The model under review builds one solid part; all positions refer to its coordinate system, in mm. A direction names the side the tool comes from. Round coordinates to 2 decimals unless told otherwise and drop trailing zeros. Write each loop counter-clockwise with the first axis right and the second up, starting at its lowest first coordinate (ties: lowest second). Pieces come first, ordered by that corner, then holes. Notation, with made-up numbers: (43.25, 26) -> (80.25, 26) arc R17 ccw to (80.25, 41) -> close; hole circle Ø3 at (21.25, -29.75). An arc over 180 degrees is marked (long way). Return JSON: item names as keys, results as strings. Group by question number.
1. Mouldability with a two-part tool opening along X and no side actions: class faces 1 (the flat face through (-3, -52, 0)), 2 (the cylindrical face through (47.69, -15.02, 24.65)), 3 (the cylindrical face through (619.984, 195.242, 747.325)) as pulls with the +X half, pulls with the -X half, needs draft (parallel to the pull), parting line crosses it, or undercut.
2. Take a section at C-C, the plane y = 0. Write out the cut boundary in (x, z), then the cut area to 3 significant figures.
3. Take a section at D-D, the plane x = -296. Write out the cut boundary in (y, z).
4. Tool access review of faces 4 (the cylindrical face through (49.205, 49.788, 747.675)), 5 (the flat face through (-88, 130, 388)), 6 (the flat face through (110, -2, 388)), 7 (the flat face through (-130, -2, 388)), 8 (the flat face through (130, -2, 388)): name each direction out of +Z, -Z, +X, -X, +Y, -Y from which nothing blocks a thin tool from reaching the whole face with its end or side.
5. Clearance check with flat-ended pins moving along their axes: P1, Ø1, axis at x = -305, y = 193.5, coming from the -Z side; P2, Ø7.5, axis at x = 88.5, z = 749, coming from the +Y side; P3, Ø7.5, axis at y = 77.5, z = 750.5, coming from the -X side. State where each tip first meets the part, or that it passes through.
6. For line 1 along Y through (x, z) = (0, 10); line 2 along X through (y, z) = (-61, 473.5), list the stretches that pass through material, from the lowest coordinate up. Write a range as from..to.
7. Take a section at A-A, the plane z = 598. Write out the cut boundary in (x, y), then the cut area to 3 significant figures.
8. Take a section at B-B, the plane x = 0. Write out the cut boundary in (y, z).
from build123d import *

# Parameters (mm, degrees)
F0_R      = 250
F1_DEPTH  = 50
F2_R      = 30
F3_W      = 260
F3_H      = 260
F3_W_2    = 220
F3_H_2    = 220
F4_DEPTH  = 685
F5_R      = 650
F5_W      = 260
F5_H      = 260
F5_W_2    = 220
F5_H_2    = 220
F6_DEPTH  = 25
F8_DEPTH  = 100
F9_W      = 160
F9_H      = 585
F10_DEPTH = 40
F11_R     = 50
F12_DEPTH = 50


with BuildPart() as f1:
    # F0 (on Top) → F1 (new body)
    with BuildSketch(Plane.XY):
        Circle(F0_R)
    extrude(amount=F1_DEPTH)

    # F2
    f2_edges = [f1.edges().sort_by_distance(p)[0] for p in [
        (-250, 0, 50),
    ]]
    fillet(f2_edges, radius=F2_R)

    # F3 (on face) → F4 (join)
    with BuildSketch(Plane.XY.offset(50)):
        Rectangle(F3_W, F3_H)
        Rectangle(F3_W_2, F3_H_2, mode=Mode.SUBTRACT)
    extrude(amount=F4_DEPTH)

    # F5 (on face) → F6 (join)
    with BuildSketch(Plane.XY.offset(735)):
        Circle(F5_R)
        Rectangle(F5_W, F5_H, mode=Mode.SUBTRACT)
        Rectangle(F5_W, F5_H)
        Rectangle(F5_W_2, F5_H_2, mode=Mode.SUBTRACT)
        Rectangle(F5_W_2, F5_H_2)
    extrude(amount=F6_DEPTH)

    # F7 (on face) → F8 (cut)
    with BuildSketch(Plane.XY.offset(760)):
        with BuildLine():
            Line((65.3834841531, 25), (96.8245836552, 25))
            ThreePointArc((96.8245836552, 25), (70.7106781187, 70.7106781187), (25, 96.8245836552))
            Line((25, 96.8245836552), (25, 65.3834841531))
            ThreePointArc((25, 65.3834841531), (49.4974746831, 49.4974746831), (65.3834841531, 25))
        make_face()
        with BuildLine():
            Line((-25, 65.3834841531), (-25, 96.8245836552))
            ThreePointArc((-25, 96.8245836552), (-70.7106781187, 70.7106781187), (-96.8245836552, 25))
            Line((-96.8245836552, 25), (-65.3834841531, 25))
            ThreePointArc((-65.3834841531, 25), (-49.4974746831, 49.4974746831), (-25, 65.3834841531))
        make_face()
        with BuildLine():
            ThreePointArc((-96.8245836552, -25), (-70.7106781187, -70.7106781187), (-25, -96.8245836552))
            Line((-25, -96.8245836552), (-25, -65.3834841531))
            ThreePointArc((-25, -65.3834841531), (-49.4974746831, -49.4974746831), (-65.3834841531, -25))
            Line((-65.3834841531, -25), (-96.8245836552, -25))
        make_face()
        with BuildLine():
            ThreePointArc((25, -96.8245836552), (70.7106781187, -70.7106781187), (96.8245836552, -25))
            Line((96.8245836552, -25), (65.3834841531, -25))
            ThreePointArc((65.3834841531, -25), (49.4974746831, -49.4974746831), (25, -65.3834841531))
            Line((25, -65.3834841531), (25, -96.8245836552))
        make_face()
    extrude(amount=-F8_DEPTH, mode=Mode.SUBTRACT)

    # F9 (on face) → F10 (cut)
    with BuildSketch(Plane(origin=(0, 130, 0), x_dir=(-1, 0, 0), z_dir=(0, 1, 0))):
        with Locations((0, 392.5)):
            Rectangle(F9_W, F9_H)
    extrude(amount=-F10_DEPTH, mode=Mode.SUBTRACT)

    # F11 (on face) → F12 (cut)
    with BuildSketch(Plane(origin=(0, 0, 0), x_dir=(1, 0, 0), z_dir=(0, 0, -1))):
        Circle(F11_R)
    extrude(amount=-F12_DEPTH, mode=Mode.SUBTRACT)


solid = f1.part
Output:
{
 "1": {"face 1": "needs draft", "face 2": "undercut", "face 3": "parting line crosses it"},
 "2": {"outline": "(-650, 735) -> (-130, 735) -> (-130, 50) -> (-220, 50) arc R30 ccw to (-250, 20) -> (-250, 0) -> (-50, 0) -> (-50, 50) -> (-110, 50) -> (-110, 735) -> (110, 735) -> (110, 50) -> (50, 50) -> (50, 0) -> (250, 0) -> (250, 20) arc R30 ccw to (220, 50) -> (130, 50) -> (130, 735) -> (650, 735) -> (650, 760) -> (-650, 760) -> close", "area": "79,500 mm^2"},
 "3": {"outline": "(-578.69, 735) -> (578.69, 735) -> (578.69, 760) -> (-578.69, 760) -> close"},
 "4": {"face 4": "+Z", "face 5": "+X, -X, +Y", "face 6": "none", "face 7": "-X, +Y, -Y", "face 8": "+X, +Y, -Y"},
 "5": {"P1": "stops at z = 735", "P2": "stops at y = 644.45", "P3": "stops at x = -645.8"},
 "6": {"line 1": "y = -250..-50, 50..250", "line 2": "x = -130..-110, 110..130"},
 "7": {"outline": "(-130, -130) -> (130, -130) -> (130, 130) -> (80, 130) -> (80, 110) -> (110, 110) -> (110, -110) -> (-110, -110) -> (-110, 110) -> (-80, 110) -> (-80, 130) -> (-130, 130) -> close", "area": "16,000 mm^2"},
 "8": {"outline": "(-650, 735) -> (-130, 735) -> (-130, 50) -> (-220, 50) arc R30 ccw to (-250, 20) -> (-250, 0) -> (-50, 0) -> (-50, 50) -> (-110, 50) -> (-110, 735) -> (110, 735) -> (110, 685) -> (130, 685) -> (130, 735) -> (650, 735) -> (650, 760) -> (-650, 760) -> close; (50, 0) -> (250, 0) -> (250, 20) arc R30 ccw to (220, 50) -> (130, 50) -> (130, 100) -> (110, 100) -> (110, 50) -> (50, 50) -> close"}
}
